Input: dimensioned drawing with shaded views. Units: mm. Origin: part minimum x, y, z. A direction names the side the tool comes from. Round coordinates to 2 decimals unless told otherwise and drop trailing zeros. Loops run counter-clockwise (first coordinate to the right, second up) from the corner with the lowest first, then second, coordinate; pieces in that order, holes last.
1) Access query for the marked faces 1 and 2. Directions: +Z, -Z, +X, -X, +Y, -Y. A direction counts if a zero-diameter tool reaches every point of the face in a straight line with its end or side. Return the directions, or none.
2) Ray query, line 1 along Y through (x, z) = (12, 2.4); line 2 along X through (y, z) = (23, 1.75); line 3 along Y through (x, z) = (7.5, 2.35). Return the intervals inside material, ascending.
3) Section B-B, the plane y = 8.5. Return loops of the section in (x, z).
4) Section D-D, the plane y = 22. Return loops of the section in (x, z).
5) Section C-C, the plane z = 1.3. Return loops of the section in (x, y).
6) Section A-A, the plane x = 12. Return loops of the section in (y, z), and give its area (3 significant figures).
7) Draft query along X for the marked faces 3, 4 and 5. Return one class per face: pulls with the +X half, pulls with the -X half, needs draft (parallel to the pull), parting line crosses it, or undercut.
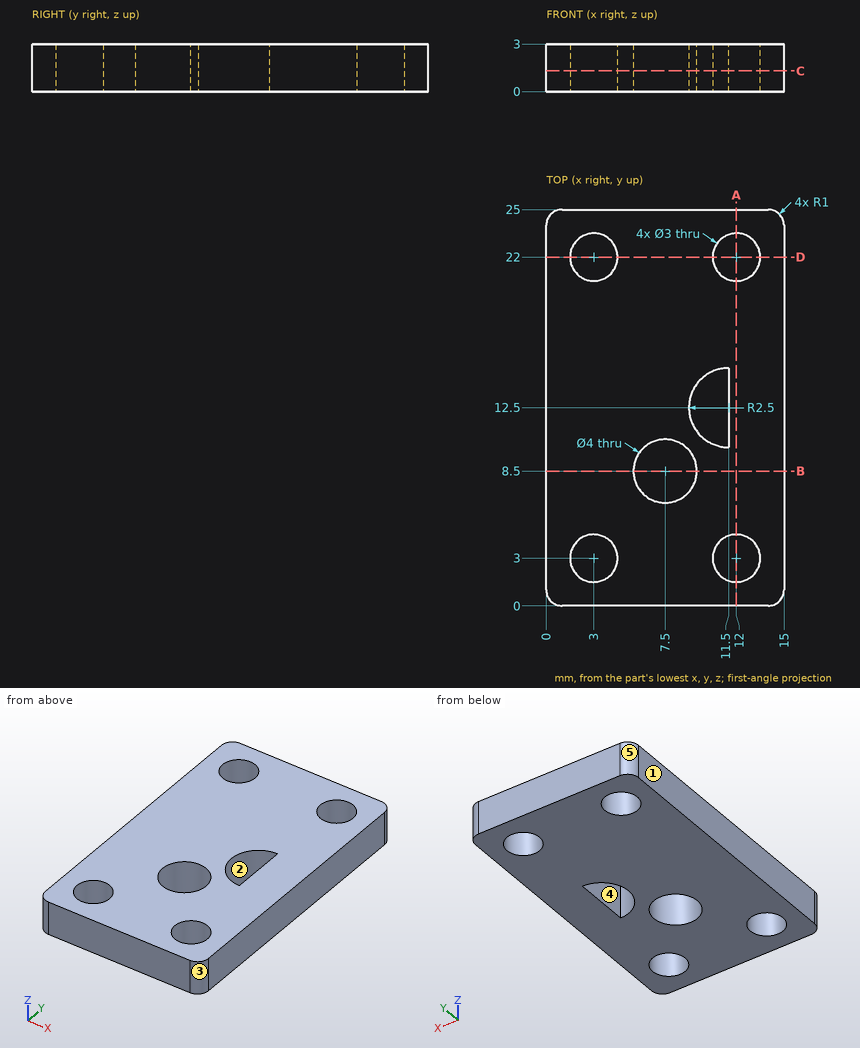
Final values:
1. face 1: +Z, -Z, -X, +Y, -Y
1. face 2: +Z, -Z
2. line 1: y = 0 to 1.5, 4.5 to 20.5, 23.5 to 25
2. line 2: x = 0 to 1.88, 4.12 to 10.88, 13.12 to 15
2. line 3: y = 0 to 6.5, 10.5 to 25
3. outline: (0, 0) - (5.5, 0) - (5.5, 3) - (0, 3) - close; (9.5, 0) - (15, 0) - (15, 3) - (9.5, 3) - close
4. outline: (0, 0) - (1.5, 0) - (1.5, 3) - (0, 3) - close; (4.5, 0) - (10.5, 0) - (10.5, 3) - (4.5, 3) - close; (13.5, 0) - (15, 0) - (15, 3) - (13.5, 3) - close
5. outline: (0, 1) arc R1 ccw to (1, 0) - (14, 0) arc R1 ccw to (15, 1) - (15, 24) arc R1 ccw to (14, 25) - (1, 25) arc R1 ccw to (0, 24) - close; hole circle Ø3 at (3, 3); hole circle Ø3 at (3, 22); hole circle Ø4 at (7.5, 8.5); hole circle Ø3 at (12, 3); hole circle Ø3 at (12, 22); hole (11.5, 10) - (11.5, 15) arc R2.5 ccw to start
6. outline: (0, 0) - (1.5, 0) - (1.5, 3) - (0, 3) - close; (4.5, 0) - (20.5, 0) - (20.5, 3) - (4.5, 3) - close; (23.5, 0) - (25, 0) - (25, 3) - (23.5, 3) - close
6. area: 57.0 mm2
7. face 3: pulls with the +X half
7. face 4: undercut
7. face 5: pulls with the -X half
